from build123d import *

# Parameters (mm, degrees)
DODANIE_WYCI_GNI_CIE1_DEPTH = 30
SZKIC2_R                    = 4
WYTNIJ_WYCI_GNI_CIE1_DEPTH  = 145.568322948
SZKIC3_R                    = 10
WYTNIJ_WYCI_GNI_CIE2_DEPTH  = 135.629120338
WYTNIJ_WYCI_GNI_CIE5_DEPTH  = 145.568323107


with BuildPart() as part:
    # Szkic1 → Dodanie-wyciągnięcie1 (new body)
    with BuildSketch(Plane.XY):
        with BuildLine():
            Line((-100, 0), (-28.575, 0))
            ThreePointArc((-28.575, 0), (0, -28.575), (28.575, 0))
            Line((28.575, 0), (100, 0))
            ThreePointArc((100, 0), (0, -100), (-100, 0))
        make_face()
    extrude(amount=DODANIE_WYCI_GNI_CIE1_DEPTH)

    # Szkic2 → Wytnij-wyciągnięcie1 (cut, through all)
    with BuildSketch(Plane(origin=(0, 0, 0), x_dir=(1, 0, 0), z_dir=(0, 1, 0))):
        with Locations(Location((-64.2875, -15, 0), (0, 0, 270))):
            Circle(SZKIC2_R)
        with Locations(Location((64.2875, -15, 0), (0, 0, 270))):
            Circle(SZKIC2_R)
    extrude(amount=-WYTNIJ_WYCI_GNI_CIE1_DEPTH, mode=Mode.SUBTRACT)

    # Szkic3 → Wytnij-wyciągnięcie2 (cut, through all)
    with BuildSketch(Plane(origin=(0, -15, 0), x_dir=(1, 0, 0), z_dir=(0, 1, 0))):
        with Locations(Location((64.2875, -15, 0), (0, 0, 270))):
            Circle(SZKIC3_R)
        with Locations(Location((-64.2875, -15, 0), (0, 0, 270))):
            Circle(SZKIC3_R)
    extrude(amount=-WYTNIJ_WYCI_GNI_CIE2_DEPTH, mode=Mode.SUBTRACT)

    # Szkic5 → Wytnij-wyciągnięcie5 (cut, through all)
    with BuildSketch(Plane(origin=(0, 0, 0), x_dir=(-1, 0, 0), z_dir=(0, 0, -1))):
        with BuildLine():
            ThreePointArc((84.486114669, -9.332546708), (80.002755588, -12.671191668), (83.234985426, -17.231865861))
            ThreePointArc((83.234985426, -17.231865861), (83.953508951, -13.296929528), (84.486114669, -9.332546708))
        make_face()
        with BuildLine():
            ThreePointArc((84.486114669, -9.332546708), (83.953508951, -13.296929528), (83.234985426, -17.231865861))
            ThreePointArc((83.234985426, -17.231865861), (86.515335048, -16.368907238), (87.953508951, -13.296929528))
            ThreePointArc((87.953508951, -13.296929528), (86.964357907, -10.663530857), (84.486114669, -9.332546708))
        make_face()
        with BuildLine():
            ThreePointArc((84.486114669, -9.332546708), (80.002755588, -12.671191668), (83.234985426, -17.231865861))
            ThreePointArc((83.234985426, -17.231865861), (83.953508951, -13.296929528), (84.486114669, -9.332546708))
        make_face()
        with BuildLine():
            ThreePointArc((84.486114669, -9.332546708), (83.953508951, -13.296929528), (83.234985426, -17.231865861))
            ThreePointArc((83.234985426, -17.231865861), (86.515335048, -16.368907238), (87.953508951, -13.296929528))
            ThreePointArc((87.953508951, -13.296929528), (86.964357907, -10.663530857), (84.486114669, -9.332546708))
        make_face()
        with BuildLine():
            ThreePointArc((42.109503339, -73.836235878), (36.773230479, -72.171528459), (34.983424582, -77.467154359))
            ThreePointArc((34.983424582, -77.467154359), (38.589192478, -75.735554556), (42.109503339, -73.836235878))
        make_face()
        with BuildLine():
            ThreePointArc((42.109503339, -73.836235878), (38.589192478, -75.735554556), (34.983424582, -77.467154359))
            ThreePointArc((34.983424582, -77.467154359), (39.477147549, -79.635751447), (42.589192478, -75.735554556))
            ThreePointArc((42.589192478, -75.735554556), (42.46741652, -74.756075981), (42.109503339, -73.836235878))
        make_face()
        with BuildLine():
            ThreePointArc((42.109503339, -73.836235878), (36.773230479, -72.171528459), (34.983424582, -77.467154359))
            ThreePointArc((34.983424582, -77.467154359), (38.589192478, -75.735554556), (42.109503339, -73.836235878))
        make_face()
        with BuildLine():
            ThreePointArc((42.109503339, -73.836235878), (38.589192478, -75.735554556), (34.983424582, -77.467154359))
            ThreePointArc((34.983424582, -77.467154359), (39.477147549, -79.635751447), (42.589192478, -75.735554556))
            ThreePointArc((42.589192478, -75.735554556), (42.46741652, -74.756075981), (42.109503339, -73.836235878))
        make_face()
        with BuildLine():
            ThreePointArc((17.231865861, -83.234985426), (12.671191668, -80.002755588), (9.332546708, -84.486114669))
            ThreePointArc((9.332546708, -84.486114669), (13.296929528, -83.953508951), (17.231865861, -83.234985426))
        make_face()
        with BuildLine():
            ThreePointArc((17.231865861, -83.234985426), (13.296929528, -83.953508951), (9.332546708, -84.486114669))
            ThreePointArc((9.332546708, -84.486114669), (13.563827184, -87.944594723), (17.296929528, -83.953508951))
            ThreePointArc((17.296929528, -83.953508951), (17.280630404, -83.592777286), (17.231865861, -83.234985426))
        make_face()
        with BuildLine():
            ThreePointArc((17.231865861, -83.234985426), (12.671191668, -80.002755588), (9.332546708, -84.486114669))
            ThreePointArc((9.332546708, -84.486114669), (13.296929528, -83.953508951), (17.231865861, -83.234985426))
        make_face()
        with BuildLine():
            ThreePointArc((17.231865861, -83.234985426), (13.296929528, -83.953508951), (9.332546708, -84.486114669))
            ThreePointArc((9.332546708, -84.486114669), (13.563827184, -87.944594723), (17.296929528, -83.953508951))
            ThreePointArc((17.296929528, -83.953508951), (17.280630404, -83.592777286), (17.231865861, -83.234985426))
        make_face()
        with BuildLine():
            ThreePointArc((-17.231865861, -83.234985426), (-13.296929528, -83.953508951), (-9.332546708, -84.486114669))
            ThreePointArc((-9.332546708, -84.486114669), (-9.305843756, -84.220406607), (-9.296929528, -83.953508951))
            ThreePointArc((-9.296929528, -83.953508951), (-12.936197864, -79.969808075), (-17.231865861, -83.234985426))
        make_face()
        with BuildLine():
            ThreePointArc((-17.231865861, -83.234985426), (-13.922667389, -87.904262313), (-9.332546708, -84.486114669))
            ThreePointArc((-9.332546708, -84.486114669), (-13.296929528, -83.953508951), (-17.231865861, -83.234985426))
        make_face()
        with BuildLine():
            ThreePointArc((-17.231865861, -83.234985426), (-13.296929528, -83.953508951), (-9.332546708, -84.486114669))
            ThreePointArc((-9.332546708, -84.486114669), (-9.305843756, -84.220406607), (-9.296929528, -83.953508951))
            ThreePointArc((-9.296929528, -83.953508951), (-12.936197864, -79.969808075), (-17.231865861, -83.234985426))
        make_face()
        with BuildLine():
            ThreePointArc((-17.231865861, -83.234985426), (-13.922667389, -87.904262313), (-9.332546708, -84.486114669))
            ThreePointArc((-9.332546708, -84.486114669), (-13.296929528, -83.953508951), (-17.231865861, -83.234985426))
        make_face()
        with BuildLine():
            ThreePointArc((-34.983424582, -77.467154359), (-36.796495821, -76.622567794), (-38.589192478, -75.735554556))
            ThreePointArc((-38.589192478, -75.735554556), (-40.360521918, -74.806605795), (-42.109503339, -73.836235878))
            ThreePointArc((-42.109503339, -73.836235878), (-40.405154477, -79.299580653), (-34.983424582, -77.467154359))
        make_face()
        with BuildLine():
            ThreePointArc((-34.589192478, -75.735554556), (-35.17863182, -73.645560297), (-36.773230479, -72.171528459))
            Line((-36.773230479, -72.171528459), (-38.589192478, -75.735554556))
            ThreePointArc((-38.589192478, -75.735554556), (-36.796495821, -76.622567794), (-34.983424582, -77.467154359))
            ThreePointArc((-34.983424582, -77.467154359), (-34.688995586, -76.623509627), (-34.589192478, -75.735554556))
        make_face()
        with BuildLine():
            Line((-38.589192478, -75.735554556), (-36.773230479, -72.171528459))
            ThreePointArc((-36.773230479, -72.171528459), (-39.780416201, -71.917048822), (-42.109503339, -73.836235878))
            ThreePointArc((-42.109503339, -73.836235878), (-40.360521918, -74.806605795), (-38.589192478, -75.735554556))
        make_face()
        with BuildLine():
            ThreePointArc((-34.589192478, -75.735554556), (-35.17863182, -73.645560297), (-36.773230479, -72.171528459))
            Line((-36.773230479, -72.171528459), (-38.589192478, -75.735554556))
            ThreePointArc((-38.589192478, -75.735554556), (-36.796495821, -76.622567794), (-34.983424582, -77.467154359))
            ThreePointArc((-34.983424582, -77.467154359), (-34.688995586, -76.623509627), (-34.589192478, -75.735554556))
        make_face()
        with BuildLine():
            Line((-38.589192478, -75.735554556), (-36.773230479, -72.171528459))
            ThreePointArc((-36.773230479, -72.171528459), (-39.780416201, -71.917048822), (-42.109503339, -73.836235878))
            ThreePointArc((-42.109503339, -73.836235878), (-40.360521918, -74.806605795), (-38.589192478, -75.735554556))
        make_face()
        with BuildLine():
            ThreePointArc((-84.486114669, -9.332546708), (-87.904262313, -13.922667389), (-83.234985426, -17.231865861))
            ThreePointArc((-83.234985426, -17.231865861), (-83.953508951, -13.296929528), (-84.486114669, -9.332546708))
        make_face()
        with BuildLine():
            ThreePointArc((-84.486114669, -9.332546708), (-83.953508951, -13.296929528), (-83.234985426, -17.231865861))
            ThreePointArc((-83.234985426, -17.231865861), (-80.881531241, -15.858755625), (-79.953508951, -13.296929528))
            ThreePointArc((-79.953508951, -13.296929528), (-81.320110279, -10.286080572), (-84.486114669, -9.332546708))
        make_face()
        with BuildLine():
            ThreePointArc((-84.486114669, -9.332546708), (-87.904262313, -13.922667389), (-83.234985426, -17.231865861))
            ThreePointArc((-83.234985426, -17.231865861), (-83.953508951, -13.296929528), (-84.486114669, -9.332546708))
        make_face()
        with BuildLine():
            ThreePointArc((-84.486114669, -9.332546708), (-83.953508951, -13.296929528), (-83.234985426, -17.231865861))
            ThreePointArc((-83.234985426, -17.231865861), (-80.881531241, -15.858755625), (-79.953508951, -13.296929528))
            ThreePointArc((-79.953508951, -13.296929528), (-81.320110279, -10.286080572), (-84.486114669, -9.332546708))
        make_face()
    extrude(amount=-WYTNIJ_WYCI_GNI_CIE5_DEPTH, mode=Mode.SUBTRACT)


solid = part.part
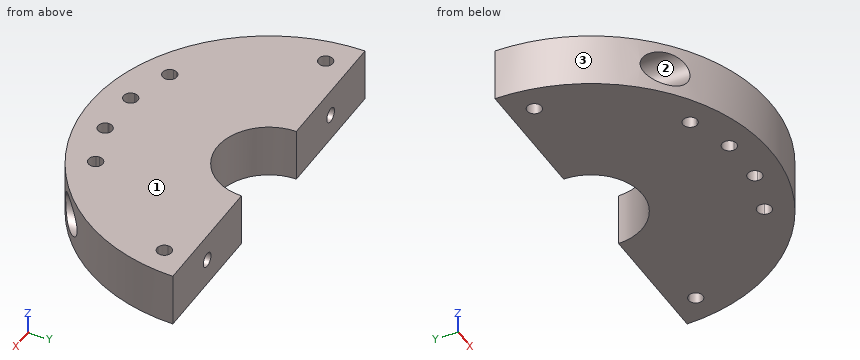
Work out the finished part from the listing and answer in its coordinate system (mm). Face numbers are marked on the shaded views. Round coordinates to 2 decimals unless told otherwise and drop trailing zeros. Loops run counter-clockwise (first coordinate to the right, second up) from the corner with the lowest first, then second, coordinate; pieces in that order, holes last. Notation, with made-up numbers: (69.25, -33) -> (80.25, -33) arc R26 ccw to (80.25, -17) -> close; hole circle Ø1 at (45.25, -38). An arc over 180 degrees is marked (long way). Use one line per item in the form item = value.
(1) Straight lines are drawn through the part: line 1 (X direction, y = -23.5, z = 10.5); line 2 (X direction, y = -8, z = 15); line 3 (X direction, y = -31, z = 15). For each, find the intervals that lie inside material, in ascending order.
Answer list:
line_1 = -97.2 to -73.22, -55.36 to -16.26, 16.26 to 55.36, 73.22 to 97.2
line_2 = -99.68 to -68.29, -60.29 to -27.43, 27.43 to 60.29, 68.29 to 99.68
line_3 = -95.07 to -74.29, -54.29 to 54.29, 74.29 to 95.07
(2) Flat-ended cylindrical pins translate along their axes: P1, Ø8, axis at x = 32, z = 8.5, coming from the -Y side; P2, Ø1.5, axis at x = 22, z = 20, coming from the -Y side; P3, Ø9, axis at x = 64.29, z = 15, coming from the -Y side. Find the tip coordinate at first contact, or state that the pin passes through.
Answer list:
P1 = -96
P2 = -97.72
P3 = -15
(3) Find section B-B on z = 9. Give the number of separate pieces and of enclosed holes in the cut face, then the cut area to 3 significant figures.
Answer list:
separate_pieces = 1
enclosed_holes = 6
area = 12,200 mm2
(4) Find section D-D on x = -77.5. Give the vertices of the cut face in (y, z).
Answer list:
outline = (-63.2, 0) -> (0, 0) -> (0, 30) -> (-63.2, 30) -> close
(5) Find section C-C on x = 0. Give the vertices of the cut face in (y, z) (3 decimals), then the cut area to 3 significant figures.
Answer list:
outline = (-100, 0) -> (-28.575, 0) -> (-28.575, 30) -> (-100, 30) -> close
area = 2,140 mm2
(6) Find section A-A on y = -52. Give the vertices of the cut face in (x, z), then the cut area to 3 significant figures.
Answer list:
outline = (-85.42, 0) -> (85.42, 0) -> (85.42, 30) -> (-85.42, 30) -> close; hole circle Ø20 at (-64.29, 15); hole circle Ø20 at (64.29, 15)
area = 4,500 mm2
(7) For a pull along X with two mould halves and no side action, classify the marked faces 1, 2 and 3 as released by +X, released by -X, zero draft, split by the parting line, or undercut.
Answer list:
face_1 = zero draft
face_2 = undercut
face_3 = split by the parting line
